Answer from the drawing. Dimensions are ordinates in mm from the lowest x, y and z of the part. Round coordinates to 2 decimals unless told otherwise and drop trailing zeros. Write each loop counter-clockwise with the first axis right and the second up, starting at its lowest first coordinate (ties: lowest second). Pieces come first, ordered by that corner, then holes. Notation, with made-up numbers: (-22.5, -3) - (36.5, -3) arc R15 cw to (36.5, 22) - close; hole circle Ø2 at (20, -11.5). An arc over 180 degrees is marked (long way). Answer in a Markdown table with one row per item.
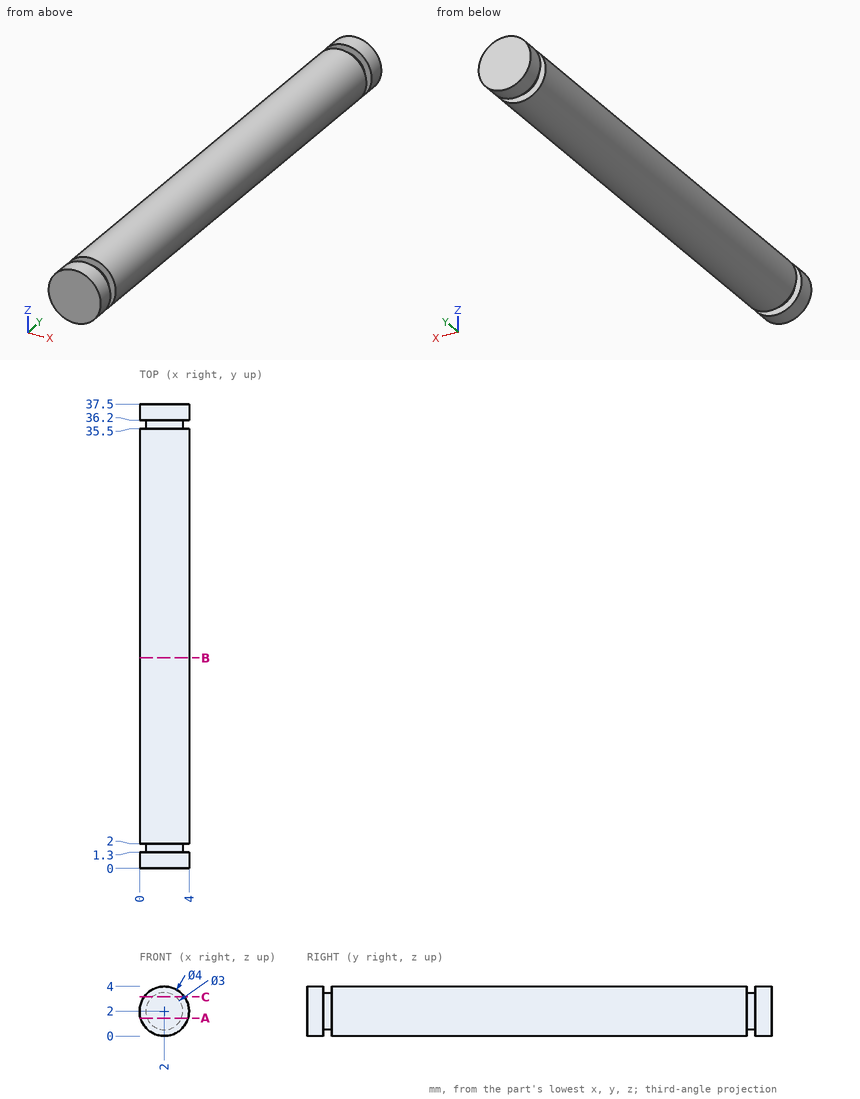
(1) Section C-C (z = 3.15) is taken. Give the vertices of the cut face in (x, y).
Checked values:
| item | result |
|---|---|
| outline | (0.36, 0) - (3.64, 0) - (3.64, 1.3) - (2.96, 1.3) - (2.96, 2) - (3.64, 2) - (3.64, 35.5) - (2.96, 35.5) - (2.96, 36.2) - (3.64, 36.2) - (3.64, 37.5) - (0.36, 37.5) - (0.36, 36.2) - (1.04, 36.2) - (1.04, 35.5) - (0.36, 35.5) - (0.36, 2) - (1.04, 2) - (1.04, 1.3) - (0.36, 1.3) - close |
(2) Section B-B (y = 17) is taken. Give the vertices of the cut face in (x, z).
Checked values:
| item | result |
|---|---|
| outline | circle Ø4 at (2, 2) |
(3) A flat-ended cylindrical pin translates along its axis: pin 1 (1 mm diameter, centred on x = 1, y = 11.5, fed in from +Z). Find the tip coordinate at first contact, or state that the pin passes through.
Checked values:
| item | result |
|---|---|
| pin 1 | stops at z = 3.94 |
(4) Find the intervals of material crossed by line 1 (Y direction, x = 3.8, z = 1.5); line 2 (X direction, y = 13.5, z = 1.9); line 3 (Z direction, x = 1.2, y = 4.5), in increasing order.
Checked values:
| item | result |
|---|---|
| line 1 | y = 0 to 1.3, 2 to 35.5, 36.2 to 37.5 |
| line 2 | x = 0 to 4 |
| line 3 | z = 0.17 to 3.83 |
(5) Section A-A (z = 1.45) is taken. Give the vertices of the cut face in (x, y).
Checked values:
| item | result |
|---|---|
| outline | (0.08, 0) - (3.92, 0) - (3.92, 1.3) - (3.4, 1.3) - (3.4, 2) - (3.92, 2) - (3.92, 35.5) - (3.4, 35.5) - (3.4, 36.2) - (3.92, 36.2) - (3.92, 37.5) - (0.08, 37.5) - (0.08, 36.2) - (0.6, 36.2) - (0.6, 35.5) - (0.08, 35.5) - (0.08, 2) - (0.6, 2) - (0.6, 1.3) - (0.08, 1.3) - close |
